Geometry: final body of the model. Coordinates: model frame, mm. A direction names the side the tool comes from. Round coordinates to 2 decimals unless told otherwise and drop trailing zeros. Loops run counter-clockwise (first coordinate to the right, second up) from the corner with the lowest first, then second, coordinate; pieces in that order, holes last. Notation, with made-up numbers: (-9, 13.5) - (5, 13.5) arc R19 cw to (5, 44.5) - close; hole circle Ø4 at (-12, 76.5). An arc over 180 degrees is marked (long way). Write item = value, one per line. Start each with the question number.
Item 1: Draft query along Z for faces 4 (the cylindrical face through (8.86, 16.38, 28.14)), 5 (the flat face through (-29, 0, -2)), 6 (the cylindrical face through (-26.36, 10.85, 5.85)). Return one class per face: pulls with the +Z half, pulls with the -Z half, needs draft (parallel to the pull), parting line crosses it, or undercut.
Item 2: First-contact query: pin 1 (10 mm diameter, centred on x = 22.5, y = 11, fed in from -Z); pin 2 (4 mm diameter, centred on x = 0, z = 7, fed in from +Y); pin 3 (16 mm diameter, centred on x = 7, z = 1, fed in from -Y); pin 4 (6 mm diameter, centred on x = 11, y = 9, fed in from +Z). Flat tips, straight axial feed; report the tip coordinate or a pass-through.
Item 3: Access query for faces 1 (the flat face through (-6, 25, 6)), 2 (the cylindrical face through (15.02, 6.48, 47.69)), 3 (the flat face through (-6, 22, -6)). Directions: +Z, -Z, +X, -X, +Y, -Y. A direction counts if a zero-diameter tool reaches every point of the face in a straight line with its end or side. Return the directions, or none.
Item 4: Section C-C (z = 33). Return loops of the section in (x, y).
Item 5: Section A-A (z = -19). Return loops of the section in (x, y), plus the area to 3 significant figures.
Item 6: Line query: line 1 (X direction, y = 24.25, z = 0); line 2 (X direction, y = 10.5, z = 0); line 3 (Y direction, x = -30.5, z = 55.5). Output: solid intervals per line, ascending. Write a range as from..to.
Item 7: Section D-D (x = 55.5). Return loops of the section in (y, z), plus the area to 3 significant figures.
Item 8: Section B-B (y = 16). Return loops of the section in (x, z).
from build123d import *

# Parameters (mm, degrees)
SKETCH_1_R          = 141.4
EXTRUDE_1_DEPTH     = 5
SKETCH_2_R          = 50
EXTRUDE_2_DEPTH     = 3
SKETCH_3_R          = 29.5
EXTRUDE_3_DEPTH     = 17
SKETCH_4_R          = 27
CUT_EXTRUDE_1_DEPTH = 22
SKETCH_5_R          = 1.5
CUT_EXTRUDE_2_DEPTH = 202.176340557


with BuildPart() as part:
    # 草图1 → 凸台-拉伸1 (new body)
    with BuildSketch(Plane(origin=(0, 0, 0), x_dir=(1, 0, 0), z_dir=(0, 1, 0))):
        with Locations(Location((0, 0, 0), (0, 0, 270))):
            Circle(SKETCH_1_R)
    extrude(amount=EXTRUDE_1_DEPTH)

    # 草图2 → 凸台-拉伸2 (add)
    with BuildSketch(Plane(origin=(0, 5, 0), x_dir=(1, 0, 0), z_dir=(0, 1, 0))):
        with Locations(Location((0, 0, 0), (0, 0, 270))):
            Circle(SKETCH_2_R)
    extrude(amount=EXTRUDE_2_DEPTH)

    # 草图3 → 凸台-拉伸3 (add)
    with BuildSketch(Plane(origin=(0, 8, 0), x_dir=(1, 0, 0), z_dir=(0, 1, 0))):
        with Locations(Location((0, 0, 0), (0, 0, 270))):
            Circle(SKETCH_3_R)
    extrude(amount=EXTRUDE_3_DEPTH)

    # 草图4 → 切除-拉伸1 (cut)
    with BuildSketch(Plane.XZ):
        with Locations(Location((0, 0, 0), (0, 0, 270))):
            Circle(SKETCH_4_R)
    extrude(amount=-CUT_EXTRUDE_1_DEPTH, mode=Mode.SUBTRACT)

    # 草图5 → 切除-拉伸2 (cut, through all)
    with BuildSketch(Plane.XZ.offset(-22)):
        with Locations(Location((0, 0, 0), (0, 0, 270))):
            Circle(SKETCH_5_R)
        with Locations(Location((0, 7, 0), (0, 0, 270))):
            Circle(SKETCH_5_R)
        with Locations(Location((7, 0, 0), (0, 0, 270))):
            Circle(SKETCH_5_R)
        with Locations(Location((0, -7, 0), (0, 0, 270))):
            Circle(SKETCH_5_R)
        with Locations(Location((-7, 0, 0), (0, 0, 270))):
            Circle(SKETCH_5_R)
    extrude(amount=-CUT_EXTRUDE_2_DEPTH, mode=Mode.SUBTRACT)


solid = part.part
Taken from the geometry:
q1.face_4 = parting line crosses it
q1.face_5 = needs draft
q1.face_6 = undercut
q2.pin_1 = -46.45
q2.pin_2 = 25
q2.pin_3 = 22
q2.pin_4 = 49.33
q3.face_1 = +Z, -Z, +X, -X, +Y
q3.face_2 = +Y
q3.face_3 = -Y
q4.outline = (-137.5, 0) - (137.5, 0) - (137.5, 5) - (37.56, 5) - (37.56, 8) - (-37.56, 8) - (-37.56, 5) - (-137.5, 5) - close
q5.outline = (-140.12, 0) - (-19.18, 0) - (-19.18, 22) - (19.18, 22) - (19.18, 0) - (140.12, 0) - (140.12, 5) - (46.25, 5) - (46.25, 8) - (22.57, 8) - (22.57, 25) - (-22.57, 25) - (-22.57, 8) - (-46.25, 8) - (-46.25, 5) - (-140.12, 5) - close
q5.area = 1,600 mm^2
q6.line_1 = -29.5..-8.5, -5.5..-1.5, 1.5..5.5, 8.5..29.5
q6.line_2 = -29.5..-27, 27..29.5
q6.line_3 = 0..5
q7.outline = (0, -130.05) - (5, -130.05) - (5, 130.05) - (0, 130.05) - close
q7.area = 1,300 mm^2
q8.outline = circle Ø59 at (0, 0); hole circle Ø54 at (0, 0)
